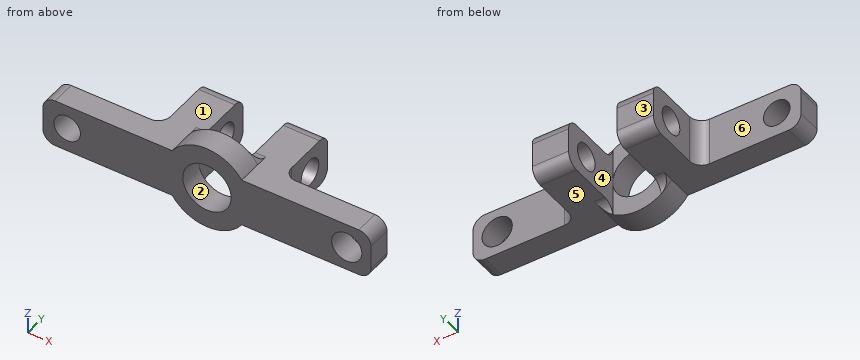
```python
from build123d import *

# Parameters (mm, degrees)
SKETCH_1_R          = 2
SKETCH_1_R_2        = 1.25
SKETCH_1_R_3        = 1.1
EXTRUDE_1_DEPTH     = 2
SKETCH_2_W          = 3
SKETCH_2_H          = 4
EXTRUDE_2_DEPTH     = 5.5
SKETCH_4_R          = 1.1
CUT_EXTRUDE_1_DEPTH = 11
FILLET_2_R          = 1
FILLET_3_R          = 1
FILLET_4_R          = 1
FILLET_5_R          = 1


with BuildPart() as part:
    # 草图1 → 凸台-拉伸1 (new body)
    with BuildSketch(Plane(origin=(0, 0, 0), x_dir=(1, 0, 0), z_dir=(0, 1, 0))):
        with BuildLine():
            Line((6.711295009, -2), (17.394013685, -2))
            Line((17.394013685, -2), (17.394013685, 2))
            Line((17.394013685, 2), (6.711295009, 2))
            ThreePointArc((6.711295009, 2), (3.839013685, 3.5), (0.966732362, 2))
            Line((0.966732362, 2), (-9.715986315, 2))
            Line((-9.715986315, 2), (-9.715986315, -2))
            Line((-9.715986315, -2), (0.966732362, -2))
            ThreePointArc((0.966732362, -2), (3.839013685, -3.5), (6.711295009, -2))
        make_face()
        with Locations(Location((3.839013685, 0, 0), (0, 0, 270))):
            Circle(SKETCH_1_R, mode=Mode.SUBTRACT)
        with Locations(Location((15.394013685, 0, 0), (0, 0, 270))):
            Circle(SKETCH_1_R_2, mode=Mode.SUBTRACT)
        with Locations(Location((-7.715986315, 0, 0), (0, 0, 270))):
            Circle(SKETCH_1_R_3, mode=Mode.SUBTRACT)
    extrude(amount=EXTRUDE_1_DEPTH)

    # 草图2 → 凸台-拉伸2 (add)
    with BuildSketch(Plane(origin=(0, 2, 0), x_dir=(1, 0, 0), z_dir=(0, 1, 0))):
        with Locations((7.339013685, 0)):
            Rectangle(SKETCH_2_W, SKETCH_2_H)
        with Locations((0.339013685, 0)):
            Rectangle(SKETCH_2_W, SKETCH_2_H)
    extrude(amount=EXTRUDE_2_DEPTH)

    # 草图4 → 切除-拉伸1 (cut)
    with BuildSketch(Plane.ZY.offset(1.160986315)):
        with Locations((0, 5.3)):
            Circle(SKETCH_4_R)
    extrude(amount=-CUT_EXTRUDE_1_DEPTH, mode=Mode.SUBTRACT)

    # 圆角2
    fillet_2_edges = [part.edges().sort_by_distance(p)[0] for p in [
        (0.339013685, 7.5, -2),
        (0.339013685, 7.5, 2),
        (7.339013685, 7.5, -2),
        (7.339013685, 7.5, 2),
    ]]
    fillet(fillet_2_edges, radius=FILLET_2_R)

    # 圆角3
    fillet_3_edges = [part.edges().sort_by_distance(p)[0] for p in [
        (-1.160986315, 2, 0),
        (8.839013685, 2, 0),
    ]]
    fillet(fillet_3_edges, radius=FILLET_3_R)

    # 圆角4
    fillet_4_edges = [part.edges().sort_by_distance(p)[0] for p in [
        (-9.715986315, 1, 2),
        (-9.715986315, 1, -2),
        (17.394013685, 1, -2),
        (17.394013685, 1, 2),
    ]]
    fillet(fillet_4_edges, radius=FILLET_4_R)

    # 圆角5
    # the kernel refuses this fillet: 1 mm, written as the material it adds along each edge
    with BuildSketch(Plane(origin=(9.211295009, 2, -2), x_dir=(0, 1, 0), z_dir=(-1, 0, 0))) as fillet_5_piece_1_section:
        with BuildLine():
            CenterArc((FILLET_5_R, FILLET_5_R), FILLET_5_R, 180, 90)
            Line((0, FILLET_5_R), (0, 0))
            Line((0, 0), (FILLET_5_R, 0))
        make_face()
    fillet_5_piece_1 = extrude(amount=3.372281323, mode=Mode.PRIVATE)
    fillet_5_piece_1 = fillet_5_piece_1 & Plane(origin=(3.839013685, 2.261416354, 0), x_dir=(0.820651806648311, 0, -0.571428571428541), z_dir=(0, -1, 0)) * Cylinder(3.5, 11, mode=Mode.PRIVATE)
    add(fillet_5_piece_1)
    with BuildSketch(Plane(origin=(1.839013685, 2, -2), x_dir=(0, 1, 0), z_dir=(-1, 0, 0))) as fillet_5_piece_2_section:
        with BuildLine():
            CenterArc((FILLET_5_R, FILLET_5_R), FILLET_5_R, 180, 90)
            Line((0, FILLET_5_R), (0, 0))
            Line((0, 0), (FILLET_5_R, 0))
        make_face()
    fillet_5_piece_2 = extrude(amount=3.372281323, mode=Mode.PRIVATE)
    fillet_5_piece_2 = fillet_5_piece_2 & Plane(origin=(3.839013685, 2.261416398, 0), x_dir=(0.820651806648311, 0, -0.571428571428541), z_dir=(0, -1, 0)) * Cylinder(3.5, 11, mode=Mode.PRIVATE)
    add(fillet_5_piece_2)
    with BuildSketch(Plane(origin=(-1.533267638, 2, 2), x_dir=(0, 0, 1), z_dir=(1, 0, 0))) as fillet_5_piece_3_section:
        with BuildLine():
            CenterArc((FILLET_5_R, -FILLET_5_R), FILLET_5_R, 90, 90)
            Line((0, -FILLET_5_R), (0, 0))
            Line((0, 0), (FILLET_5_R, 0))
        make_face()
    fillet_5_piece_3 = extrude(amount=3.372281323, mode=Mode.PRIVATE)
    fillet_5_piece_3 = fillet_5_piece_3 & Plane(origin=(3.839013685, 2.26141635, 0), x_dir=(-0.8206518066482962, 0, 0.5714285714285624), z_dir=(0, -1, 0)) * Cylinder(3.5, 11, mode=Mode.PRIVATE)
    add(fillet_5_piece_3)
    with BuildSketch(Plane(origin=(5.839013685, 2, 2), x_dir=(0, 1, 0), z_dir=(1, 0, 0))) as fillet_5_piece_4_section:
        with BuildLine():
            CenterArc((FILLET_5_R, FILLET_5_R), FILLET_5_R, 180, 90)
            Line((0, FILLET_5_R), (0, 0))
            Line((0, 0), (FILLET_5_R, 0))
        make_face()
    fillet_5_piece_4 = extrude(amount=3.372281323, mode=Mode.PRIVATE)
    fillet_5_piece_4 = fillet_5_piece_4 & Plane(origin=(3.839013685, 2.261416398, 0), x_dir=(-0.8206518066482962, 0, 0.5714285714285624), z_dir=(0, -1, 0)) * Cylinder(3.5, 11, mode=Mode.PRIVATE)
    add(fillet_5_piece_4)


solid = part.part
```
CAD build for the part. Positions are in the model's coordinates, mm. Face numbers are marked on the shaded views. A direction names the side the tool comes from. Coordinates: 2 decimals unless noted, no trailing zeros. Write each loop counter-clockwise with the first axis right and the second up, starting at its lowest first coordinate (ties: lowest second). Pieces come first, ordered by that corner, then holes.
(1) Cut at A-A, the plane y = 6. List the corners of the cut face in (x, z).
(2) Cut at C-C, the plane y = 1.5. List the corners of the cut face in (x, z).
(3) Cut at D-D, the plane x = 4.75. List the corners of the cut face in (y, z), and give its area (3 significant figures).
(4) 3-axis set-ups, long thin cutter, end or side, ignore diameter. For the marked faces 4, 5 and 6: which of +Z, -Z, +X, -X, +Y, -Y reach the whole face in a straight line?
(5) Cut at B-B, the plane z = 0.25. Count the separate pieces of the cut face and the enclosed holes in it, and give its area (3 significant figures).
(6) Two-plate mould, pull along Z, no slides. Class the marked faces 1, 2 and 3: +Z half, -Z half, draft (parallel to the pull), parting line (faces both ways), or undercut.
(7) Drill centre lines: probe 1 along X at (y, z) = (0.85, 0); probe 2 along X at (y, z) = (4.75, -1.75); probe 3 along X at (y, z) = (1.75, -1). Where is each one in solid material? Low to high.
(8) Flat gauge pins, fed straight in: pin 1 (3 mm diameter, centred on x = -3.5, y = 1, fed in from -Z); pin 2 (2 mm diameter, centred on x = 13, z = 1, fed in from +Y); pin 3 (2.5 mm diameter, centred on x = -7.72, z = 0, fed in from -Y); pin 4 (2 mm diameter, centred on y = 5.5, z = -1, fed in from +X). Where does each tip first touch, or does it go through?
Geometry says:
1. outline: (-1.16, -2) - (1.84, -2) - (1.84, -0.85) - (-1.16, -0.85) - close; (-1.16, 0.85) - (1.84, 0.85) - (1.84, 2) - (-1.16, 2) - close; (5.84, -2) - (8.84, -2) - (8.84, -0.85) - (5.84, -0.85) - close; (5.84, 0.85) - (8.84, 0.85) - (8.84, 2) - (5.84, 2) - close
2. outline: (-9.72, -1) arc R1 ccw to (-8.72, -2) - (0.97, -2) arc R3.5 ccw to (6.71, -2) - (16.39, -2) arc R1 ccw to (17.39, -1) - (17.39, 1) arc R1 ccw to (16.39, 2) - (6.71, 2) arc R3.5 ccw to (0.97, 2) - (-8.72, 2) arc R1 ccw to (-9.72, 1) - close; hole circle Ø2.2 at (-7.72, 0); hole circle Ø4 at (3.84, 0); hole circle Ø2.5 at (15.39, 0)
3. outline: (0, -3.38) - (2, -3.38) - (2, -1.78) - (0, -1.78) - close; (0, 1.78) - (2, 1.78) - (2, 3.38) - (0, 3.38) - close
3. area: 6.40 mm2
4. face 4: +Z, -Z, +Y
4. face 5: -Z, +X, +Y
4. face 6: +Z, -Z, -X, +Y
5. separate pieces: 6
5. enclosed holes: 0
5. area: 57.7 mm2
6. face 1: +Z half
6. face 2: undercut
6. face 3: draft
7. probe 1: x = -9.72 to -8.82, -6.62 to 1.84, 5.84 to 14.14, 16.64 to 17.39
7. probe 2: x = -1.16 to 1.84, 5.84 to 8.84
7. probe 3: x = -9.72 to -8.17, -7.26 to 2.11, 5.57 to 14.64, 16.14 to 17.39
8. pin 1: stops at z = -2
8. pin 2: stops at y = 2
8. pin 3: stops at y = 0
8. pin 4: stops at x = 8.84
